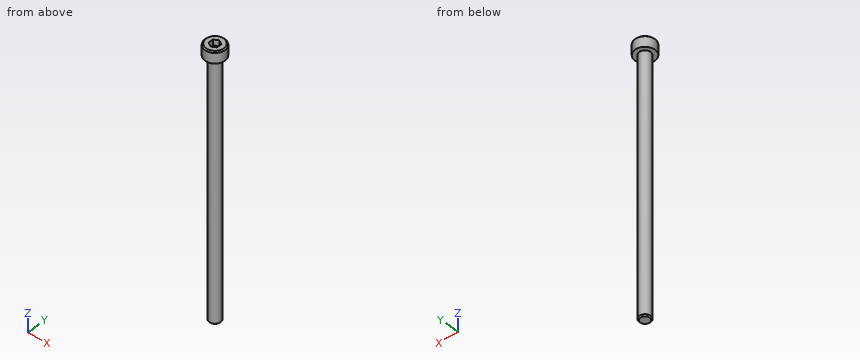
Autodesk Inventor part; units mm, degrees
ref_plane "YZ Plane" through (0, 0, 0) normal (1, 0, 0) x (0, 1, 0)
ref_plane "XZ Plane" through (0, 0, 0) normal (0, 1, 0) x (-1, 0, 0)
ref_plane "XY Plane" through (0, 0, 0) normal (0, 0, 1) x (1, 0, 0)
sketch "Sketch1" plane through (0, 0, 0) normal (0, 0, 1) x (1, 0, 0)
  circle A0 centre (0, 0) radius 2
  dimension "Diameter" = 4
extrude "Extrusion1" add sketch "Sketch1" along normal blind 90
sketch "Sketch2" plane through (0, 0, 90) normal (0, 0, 1) x (1, 0, 0)
  circle A0 centre (0, 0) radius 2
  circle A1 centre (0, 0) radius 3.5
  dimension "Head_Diameter" = 7
extrude "Extrusion2" add sketch "Sketch2" along normal blind 4 contours A0 | A1
sketch "Sketch3" plane through (0, 0, 94) normal (0, 0, 1) x (1, 0, 0)
  circle A0 centre (0, 0) radius 3.5
  circle A1 centre (0, 0) radius 1.7321 construction
  line L0 (0, 1.7321) -> (1.5, 0.866)
  line L1 (1.5, -0.866) -> (1.5, 0.866)
  line L2 (0, 1.7321) -> (-1.5, 0.866)
  line L3 (-1.5, -0.866) -> (-1.5, 0.866)
  line L4 (-1.5, -0.866) -> (0, -1.7321)
  line L5 (1.5, -0.866) -> (0, -1.7321)
  dimension "Hex_Width" = 3
extrude "Extrusion3" cut sketch "Sketch3" against normal blind 2 contours L0 L1 L5 L4 L3 L2
thread "Thread1"
chamfer "Chamfer1" distance 0.4 angle 45 2 edges at (-3.5, 0, 94) (-2, 0, 0)
equation "\"d9\" = ThreadLength"
equation "\"d12\" = Chamfer"
equation "\"ThreadLength\" = 20"
properties part number "SCREW, SOCKET HD, P, 12_9, M4X0_7X90" material "Steel, MS"
Here's how the part is built. I have some questions about the finished solid (model axes, mm). Round coordinates to 2 decimals unless told otherwise and drop trailing zeros. Loops run counter-clockwise (first coordinate to the right, second up) from the corner with the lowest first, then second, coordinate; pieces in that order, holes last.
1. Suppose I cut it at A-A, the plane y = 0. Please give me the cut outline in (x, z), and give its area (3 significant figures).
Answers:
outline: (-3.5, 90) - (-2, 90) - (-2, 0.4) - (-1.6, 0) - (1.6, 0) - (2, 0.4) - (2, 90) - (3.5, 90) - (3.5, 93.6) - (3.1, 94) - (1.5, 94) - (1.5, 92) - (-1.5, 92) - (-1.5, 94) - (-3.1, 94) - (-3.5, 93.6) - close
area: 382 mm2
2. Will these pins go through, and if not, where does the flat tip stop? pin 1 (0.5 mm diameter, centred on y = -0.5, z = 93, fed in from +X); pin 2 (4 mm diameter, centred on x = -0.5, z = 82.5, fed in from -Y); pin 3 (4 mm diameter, centred on y = -2.5, z = 58.5, fed in from -X).
Answers:
pin 1: stops at x = 3.49
pin 2: stops at y = -2
pin 3: stops at x = -1.94
3. If I drill on probe 1 along X at (y, z) = (-1, 51); probe 2 along Z at (x, y) = (0.5, 2.5); probe 3 along Z at (x, y) = (0.75, 0), over which ranges is the centre line in solid material (lowest first)?
Answers:
probe 1: x = -1.73 to 1.73
probe 2: z = 90 to 94
probe 3: z = 0 to 92
4. Suppose I cut it at B-B, the plane z = 19. Please give me the cut outline in (x, y).
Answers:
outline: circle Ø4 at (0, 0)
